from build123d import *

# Parameters (mm, degrees)
SKETCH1_R           = 150
SKETCH1_R_2         = 40
BOSS_EXTRUDE1_DEPTH = 10
SKETCH2_R           = 25
BOSS_EXTRUDE2_DEPTH = 100
SKETCH3_R           = 15
BOSS_EXTRUDE3_DEPTH = 20
SKETCH4_W           = 102.125411964
SKETCH4_H           = 75.272699472
BOSS_EXTRUDE4_DEPTH = 20


with BuildPart() as part:
    # Sketch1 → Boss-Extrude1 (new body)
    with BuildSketch(Plane.XY):
        Circle(SKETCH1_R)
        with Locations((0, 95)):
            Circle(SKETCH1_R_2, mode=Mode.SUBTRACT)
        with Locations((95, 0)):
            Circle(SKETCH1_R_2, mode=Mode.SUBTRACT)
        with Locations((0, -95)):
            Circle(SKETCH1_R_2, mode=Mode.SUBTRACT)
        with Locations((-95, 0)):
            Circle(SKETCH1_R_2, mode=Mode.SUBTRACT)
    extrude(amount=BOSS_EXTRUDE1_DEPTH)

    # Sketch2 → Boss-Extrude2 (add)
    with BuildSketch(Plane(origin=(0, 0, 0), x_dir=(-1, 0, 0), z_dir=(0, 0, -1))):
        Circle(SKETCH2_R)
    extrude(amount=BOSS_EXTRUDE2_DEPTH)

    # Sketch3 → Boss-Extrude3 (add)
    with BuildSketch(Plane(origin=(0, 0, -100), x_dir=(-1, 0, 0), z_dir=(0, 0, -1))):
        Circle(SKETCH3_R)
    extrude(amount=BOSS_EXTRUDE3_DEPTH)

    # Sketch4 → Boss-Extrude4 (add)
    with BuildSketch(Plane(origin=(0, 0, -120), x_dir=(-1, 0, 0), z_dir=(0, 0, -1))):
        Rectangle(SKETCH4_W, SKETCH4_H)
    extrude(amount=BOSS_EXTRUDE4_DEPTH)


solid = part.part
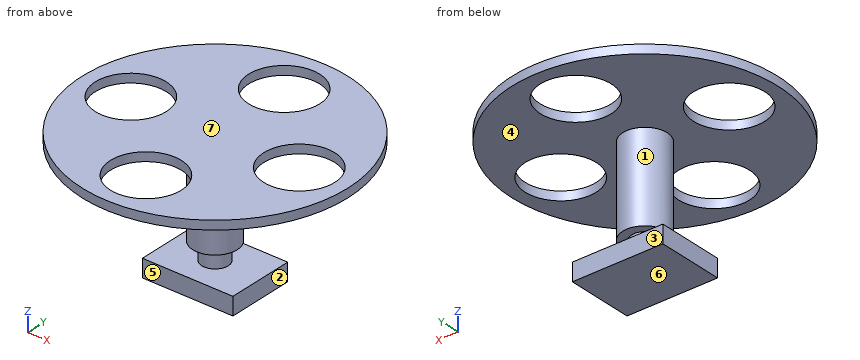
Could you check a few things on this model? Use its own coordinates, in mm. Face numbers are marked on the shaded views. A direction names the side the tool comes from. Give positions to 0.01 mm unless a question says otherwise; leave off trailing zeros. Order: outer loops, then holes, each group sorted by start corner. A loop starts at its lowest first (then second) coordinate and runs counter-clockwise, first axis right, second up. Notation, with made-up numbers: (18.5, 69) - (43.5, 69) arc R33 cw to (43.5, 106) - close; hole circle Ø4 at (79.25, 12.5). An arc over 180 degrees is marked (long way). Return JSON: item names as keys, results as strings. Group by question number.
Q1. Please list where these lines run through material, in increasing order: line 1 along Y through (x, z) = (0, 8); line 2 along Z through (x, y) = (14.5, -7.5); line 3 along X through (y, z) = (18.5, 4.5). Write a range as [from, to].
Q2. Which directions (+Z, -Z, +X, -X, +Y, -Y) give clear straight access to the entire face, cutting with the end or side of a thin tool? Please do the marked faces 1, 2 and 3.
Q3. Suppose I cut it at A-A, the plane x = 0. Please give me the cut outline in (y, z).
Q4. Will these pins go through, and if not, where does the flat tip stop? pin 1 Ø6 at (y, z) = (3.5, -130) entering from -X; pin 2 Ø10 at (x, z) = (22, -134) entering from +Y; pin 3 Ø6 at (x, y) = (71.5, 44.5) entering from -Z.
Q5. Suppose I cut it at B-B, the plane y = -95. Please give me the cut outline in (x, z).
Q6. Thinking about a two-plate mould opening in Z: for the marked faces 4, 5, 6 and 7, which applies, pulls with the +Z half, pulls with the -Z half, needs draft (parallel to the pull), parting line crosses it, or undercut?
Q7. Suppose I cut it at C-C, the plane x = -113.5. Please give me the cut outline in (y, z), and give its area (3 significant figures).
Q8. Suppose I cut it at D-D, the plane y = 31. Please give me the cut outline in (x, z), and give its area (3 significant figures).
Resolved:
{
 "1": {"line 1": "y = [-150, -135], [-55, 55], [135, 150]", "line 2": "z = [-140, -120], [-100, 10]", "line 3": "x = [-148.85, -130.46], [-59.54, 59.54], [130.46, 148.85]"},
 "2": {"face 1": "none", "face 2": "-Z, +X, +Y, -Y", "face 3": "-Z, +X, -X, +Y"},
 "3": {"outline": "(-150, 0) - (-135, 0) - (-135, 10) - (-150, 10) - close; (-55, 0) - (-25, 0) - (-25, -100) - (-15, -100) - (-15, -120) - (-37.64, -120) - (-37.64, -140) - (37.64, -140) - (37.64, -120) - (15, -120) - (15, -100) - (25, -100) - (25, 0) - (55, 0) - (55, 10) - (-55, 10) - close; (135, 0) - (150, 0) - (150, 10) - (135, 10) - close"},
 "4": {"pin 1": "stops at x = -51.06", "pin 2": "stops at y = 37.64", "pin 3": "stops at z = 0"},
 "5": {"outline": "(-116.08, 0) - (-40, 0) - (-40, 10) - (-116.08, 10) - close; (40, 0) - (116.08, 0) - (116.08, 10) - (40, 10) - close"},
 "6": {"face 4": "undercut", "face 5": "needs draft", "face 6": "pulls with the -Z half", "face 7": "pulls with the +Z half"},
 "7": {"outline": "(-98.07, 0) - (-35.46, 0) - (-35.46, 10) - (-98.07, 10) - close; (35.46, 0) - (98.07, 0) - (98.07, 10) - (35.46, 10) - close", "area": "1,250 mm2"},
 "8": {"outline": "(-146.76, 0) - (-120.28, 0) - (-120.28, 10) - (-146.76, 10) - close; (-69.72, 0) - (69.72, 0) - (69.72, 10) - (-69.72, 10) - close; (-51.06, -140) - (51.06, -140) - (51.06, -120) - (-51.06, -120) - close; (120.28, 0) - (146.76, 0) - (146.76, 10) - (120.28, 10) - close", "area": "3,970 mm2"}
}
